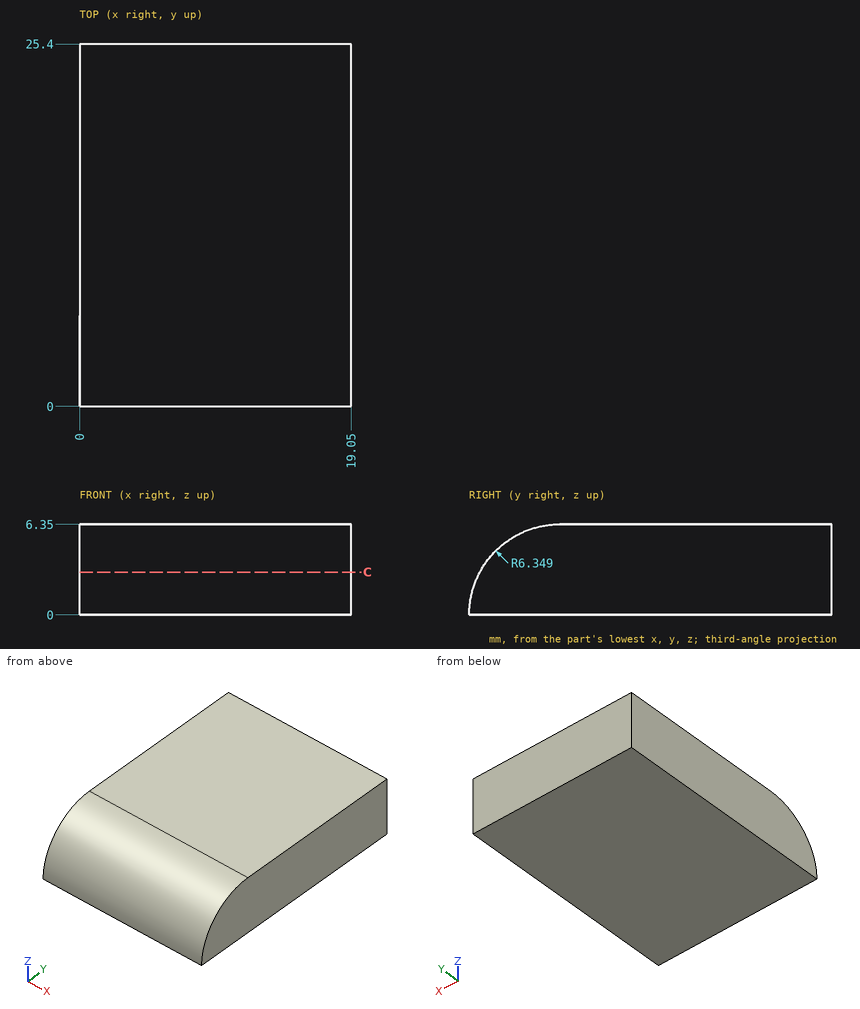
Here's the drawing with two shaded views (mm, measured from the low corner). I have some questions. Round coordinates to 2 decimals unless told otherwise and drop trailing zeros. Order: outer loops, then holes, each group sorted by start corner. A loop starts at its lowest first (then second) coordinate and runs counter-clockwise, first axis right, second up. Notation, with made-up numbers: (-12, 38) -> (-5, 38) arc R21 ccw to (-5, 76) -> close; hole circle Ø4 at (27, 84.5). An arc over 180 degrees is marked (long way). Use a Markdown table: item, result. Add a question column.
(1) For pin 1 Ø3 at (x, y) = (11, 4.5) entering from +Z; pin 2 Ø1.5 at (x, z) = (15.5, 2) entering from -Y, each with a flat end and sliding along its axis, tell me the tip position at first contact or that it passes through.
(2) I need wall thicknesses on line 1 along Y through (x, z) = (16.25, 3.5); line 2 along Y through (x, z) = (3, 2.25); line 3 along Z through (x, y) = (15.25, 6.25). Which ranges of each line are inside material? Lowest first, please.
(3) Suppose I cut it at C-C, the plane z = 3. Please give me the cut outline in (x, y).
Verdict:
| question | item | result |
|---|---|---|
| 1 | pin 1 | z = 6.34 |
| 1 | pin 2 | y = 0.12 |
| 2 | line 1 | 1.05 to 25.4 |
| 2 | line 2 | 0.41 to 25.4 |
| 2 | line 3 | 0 to 6.35 |
| 3 | outline | (0, 0.75) -> (19.05, 0.75) -> (19.05, 25.4) -> (0, 25.4) -> close |
